```python
from build123d import *

# Parameters (mm, degrees)
F0_W     = 50.8
F0_H     = 50.8
F1_DEPTH = 101.6
F2_SIZE  = 6.35


with BuildPart() as f1:
    # F0 (on Front) → F1 (new body)
    with BuildSketch(Plane.XZ):
        Polygon((50.8, -203.2), (50.8, 609.6), (-50.8, 609.6), (-50.8, 406.4), (-50.8, -203.2), (-50.8, -609.6), (50.8, -609.6), align=None)
        with Locations((0, -203.2)):
            Rectangle(F0_W, F0_H, mode=Mode.SUBTRACT)
        with Locations((0, 406.4)):
            Rectangle(F0_W, F0_H, mode=Mode.SUBTRACT)
    extrude(amount=F1_DEPTH)

    # F2
    f2_edges = [f1.edges().sort_by_distance(p)[0] for p in [
        (-50.8, -101.6, 0),
        (50.8, -101.6, 0),
        (50.8, 0, 0),
        (-50.8, 0, 0),
        (0, 0, 609.6),
        (50.8, -50.8, 609.6),
        (0, -101.6, 609.6),
        (-50.8, -50.8, 609.6),
    ]]
    chamfer(f2_edges, length=F2_SIZE)


solid = f1.part
```
Geometry: final body of the model. Coordinates: model frame, mm. A direction names the side the tool comes from. Give positions to 0.01 mm unless a question says otherwise; leave off trailing zeros. Order: outer loops, then holes, each group sorted by start corner. A loop starts at its lowest first (then second) coordinate and runs counter-clockwise, first axis right, second up. Notation, with made-up numbers: (7.25, 80) -> (44.25, 80) arc R7 ccw to (44.25, 93) -> close; hole circle Ø4 at (52.5, 18). An arc over 180 degrees is marked (long way). Write each question's results on one line, items separated by ' | '. Start each with the question number.
1) Section B-B (x = -4). Return loops of the section in (y, z).
2) Set-up query: faces 1 (the flat face through (-25.4, -50, 406)), 2 (the flat face through (-1, -101.6, 5)). Return all of +Z, -Z, +X, -X, +Y, -Y with unobstructed straight access to the full face (end or side cutting, diameter ignored); none if empty.
3) Draft query along Z for faces 3 (the flat face through (-25.4, -50, -204)), 4 (the flat face through (1, -50, 609.6)), 5 (the flat face through (50.8, -50, -12)), 6 (the flat face through (0, -50, 381)). Return one class per face: pulls with the +Z half, pulls with the -Z half, needs draft (parallel to the pull), parting line crosses it, or undercut.
4) Line query: line 1 (Z direction, x = 1.5, y = -27.5); line 2 (X direction, y = -67.5, z = -196); line 3 (Y direction, x = -45, z = 20). Output: solid intervals per line, ascending. Write a range as from..to.
5) Section A-A (y = -59). Return loops of the section in (x, z), then the cut area to 3 significant figures.
Calculated:
1) outline: (-101.6, -609.6) -> (0, -609.6) -> (0, -228.6) -> (-101.6, -228.6) -> close; (-101.6, -177.8) -> (0, -177.8) -> (0, 381) -> (-101.6, 381) -> close; (-101.6, 431.8) -> (0, 431.8) -> (0, 603.25) -> (-6.35, 609.6) -> (-95.25, 609.6) -> (-101.6, 603.25) -> close
2) face 1: +Y, -Y | face 2: +Z, -Z, +X, -X, -Y
3) face 3: undercut | face 4: pulls with the +Z half | face 5: needs draft | face 6: undercut
4) line 1: -609.6..-228.6, -177.8..381, 431.8..609.6 | line 2: -50.8..-25.4, 25.4..50.8 | line 3: -101.05..-0.55
5) outline: (-50.8, -609.6) -> (50.8, -609.6) -> (50.8, 603.25) -> (44.45, 609.6) -> (-44.45, 609.6) -> (-50.8, 603.25) -> close; hole (-25.4, -228.6) -> (25.4, -228.6) -> (25.4, -177.8) -> (-25.4, -177.8) -> close; hole (-25.4, 381) -> (25.4, 381) -> (25.4, 431.8) -> (-25.4, 431.8) -> close | area: 119,000 mm2
